from build123d import *

# Parameters (mm, degrees)
BOSS_EXTRUDE1_DEPTH        = 40
SKETCH2_R                  = 2.75
CUT_EXTRUDE1_DEPTH         = 53.048054719
F_5_0_5_5_DIAMETER_HOLE1_D = 5.5


with BuildPart() as part:
    # Sketch1 → Boss-Extrude1 (new body)
    with BuildSketch(Plane.XY):
        Polygon((0, 0), (0, 25), (-3, 25), (-3, 3), (-25, 3), (-25, 0), align=None)
    extrude(amount=BOSS_EXTRUDE1_DEPTH)

    # Sketch2 → Cut-Extrude1 (cut, through all)
    with BuildSketch(Plane(origin=(0, 3, 0), x_dir=(1, 0, 0), z_dir=(0, 1, 0))):
        with Locations(Location((-15, -10, 0), (0, 0, 180))):
            Circle(SKETCH2_R)
        with Locations((-15, -30)):
            Circle(SKETCH2_R)
    extrude(amount=-CUT_EXTRUDE1_DEPTH, mode=Mode.SUBTRACT)

    # Ø5.0 (5.5) Diameter Hole1 (through all)
    with Locations(Plane.ZY.offset(3)):
        with Locations((20, 15)):
            Hole(F_5_0_5_5_DIAMETER_HOLE1_D / 2)


solid = part.part
Build history of the part. All positions in model axes, mm. A direction names the side the tool comes from. Give positions to 0.01 mm unless a question says otherwise; leave off trailing zeros. Order: outer loops, then holes, each group sorted by start corner. A loop starts at its lowest first (then second) coordinate and runs counter-clockwise, first axis right, second up. Notation, with made-up numbers: M 85,5.25 L 96,5.25 A28 cw 96,24.25 Z; hole C 89.25,3 d9. An arc over 180 degrees is marked long. Put each result on its own line as item: value.
Item 1: Slice it at C-C, the plane z = 20. Write the cut outline in (x, y), plus the area to 4 significant figures.
From the geometry:
outline: M -25,0 L 0,0 L 0,12.25 L -3,12.25 L -3,3 L -25,3 Z; M -3,17.75 L 0,17.75 L 0,25 L -3,25 Z
area: 124.5 mm2
Item 2: Slice it at B-B, the plane y = 15. Write the cut outline in (x, z), plus the area to 4 significant figures.
From the geometry:
outline: M -3,0 L 0,0 L 0,17.25 L -3,17.25 Z; M -3,22.75 L 0,22.75 L 0,40 L -3,40 Z
area: 103.5 mm2
Item 3: 3-axis set-ups, long thin cutter, end or side, ignore diameter. For faces 1 (the flat face through (-3, 12, 20)), 2 (the cylindrical face through (-12.973, 1.521, 11.859)): which of +Z, -Z, +X, -X, +Y, -Y reach the whole face in a straight line?
From the geometry:
face 1: +Z, -Z, -X, +Y
face 2: +Y, -Y
Item 4: Slice it at A-A, the plane x = -15. Write the cut outline in (y, z).
From the geometry:
outline: M 0,0 L 3,0 L 3,7.25 L 0,7.25 Z; M 0,12.75 L 3,12.75 L 3,27.25 L 0,27.25 Z; M 0,32.75 L 3,32.75 L 3,40 L 0,40 Z
Item 5: Slice it at D-D, the plane z = 6. Write the cut outline in (x, y).
From the geometry:
outline: M -25,0 L 0,0 L 0,25 L -3,25 L -3,3 L -25,3 Z
Item 6: Flat gauge pins, fed straight in: pin 1 Ø3 at (x, y) = (-5, 9.5) entering from -Z; pin 2 Ø10 at (x, z) = (-2.5, 15.5) entering from -Y; pin 3 Ø2 at (y, z) = (12.5, 30.5) entering from -X; pin 4 Ø7 at (x, z) = (-15, 30) entering from +Y. Where does each tip first touch, or does it go through?
From the geometry:
pin 1: passes through
pin 2: stops at y = 0
pin 3: stops at x = -3
pin 4: stops at y = 3
Item 7: Two-plate mould, pull along Z, no slides. Class faces 3 (the cylindrical face through (-1.479, 15.121, 22.747)), 4 (the flat face through (-7, 2, 40)), 5 (the flat face through (-25, 2, 20)): +Z half, -Z half, draft (parallel to the pull), parting line (faces both ways), or undercut.
From the geometry:
face 3: undercut
face 4: +Z half
face 5: draft
Item 8: Probe line 1 (X direction, y = 2.05, z = 30); line 2 (Z direction, x = -15, y = 2); line 3 (X direction, y = 18, z = 20). List the from-to ranges inside material, lowest first. Write a range as [from, to].
From the geometry:
line 1: x = [-25, -17.75], [-12.25, 0]
line 2: z = [0, 7.25], [12.75, 27.25], [32.75, 40]
line 3: x = [-3, 0]
